from build123d import *

# Parameters (mm, degrees)
SKETCH2_W           = 29.3
SKETCH2_H           = 18.3
BOSS_EXTRUDE1_DEPTH = 1.6
SKETCH3_R           = 4
BOSS_EXTRUDE2_DEPTH = 1
SKETCH4_R           = 3.125
BOSS_EXTRUDE3_DEPTH = 1.6
SKETCH5_R           = 3.9
BOSS_EXTRUDE4_DEPTH = 8.5


with BuildPart() as part:
    # Sketch2 → Boss-Extrude1 (new body)
    with BuildSketch(Plane(origin=(0, 0, 0), x_dir=(1, 0, 0), z_dir=(0, 1, 0))):
        with Locations((14.65, 9.15)):
            Rectangle(SKETCH2_W, SKETCH2_H)
    extrude(amount=BOSS_EXTRUDE1_DEPTH)

    # Sketch3 → Boss-Extrude2 (add)
    with BuildSketch(Plane(origin=(29.3, 0, 0), x_dir=(0, 0, -1), z_dir=(1, 0, 0))):
        with Locations((12.6, 2.1)):
            Circle(SKETCH3_R)
    extrude(amount=BOSS_EXTRUDE2_DEPTH)

    # Sketch4 → Boss-Extrude3 (add)
    with BuildSketch(Plane(origin=(30.3, 0, 0), x_dir=(0, 0, -1), z_dir=(1, 0, 0))):
        with Locations((12.6, 2.1)):
            Circle(SKETCH4_R)
    extrude(amount=BOSS_EXTRUDE3_DEPTH)

    # Sketch5 → Boss-Extrude4 (add)
    with BuildSketch(Plane(origin=(31.9, 0, 0), x_dir=(0, 0, -1), z_dir=(1, 0, 0))):
        with Locations((12.6, 2.1)):
            Circle(SKETCH5_R)
    extrude(amount=BOSS_EXTRUDE4_DEPTH)


solid = part.part
Design review of the part built by this model. Coordinates are the model's own, in mm. A direction names the side the tool comes from. Round coordinates to 2 decimals unless told otherwise and drop trailing zeros. Write each loop counter-clockwise with the first axis right and the second up, starting at its lowest first coordinate (ties: lowest second). Pieces come first, ordered by that corner, then holes. Notation, with made-up numbers: M 59,81 L 74,81 A24 ccw 74,91 Z; hole C 14,15 d3. An arc over 180 degrees is marked long. One line per item, written item: value. Start each with the question number.
1. Take a section at B-B on y = 2.1. State the section outline as (x, z) points (3 decimals), then the cut area to 3 significant figures.
2. Take a section at C-C on x = 26. State the section outline as (y, z) points.
3. Take a section at D-D on x = 33. State the section outline as (y, z) points, then the cut area to 3 significant figures.
4. To check wall thickness, follow probe 1 along X at (y, z) = (3.5, -15.5); probe 2 along Y at (x, z) = (7.5, -8.5); probe 3 along X at (y, z) = (4.5, -12). State the ranges of each line that lie inside material, in increasing order. Write a range as from..to.
5. For faces 4 (the face through (36.09, 2.271, -8.704)), 5 (the face through (14, 1.6, -9)), 6 (the face through (31.9, 0, -10)), 7 (the face through (29.3, -1, -13)), list the 3-axis set-ups (+Z, -Z, +X, -X, +Y, -Y) from which the entire face can be reached by the end or side of a thin tool; tool diameter is ignored.
6. Draft analysis for pull direction X (two halves, no side actions). For faces 1 (the face through (30.3, 0, -10)), 2 (the face through (14, 0, -9)), 3 (the face through (29.3, 3, -13)), state which applies: pulls with the +X half, pulls with the -X half, needs draft (parallel to the pull), parting line crosses it, or undercut.
7. Clearance check with flat-ended pins moving along their axes: P1, Ø1.5, axis at y = -1, z = -14.5, coming from the -X side; P2, Ø2, axis at x = 6.5, z = -5, coming from the -Y side; P3, Ø0.5, axis at y = 0.5, z = -3.5, coming from the +X side. State where each tip first meets the part, or that it passes through.
8. Take a section at A-A on z = -12.6. State the section outline as (x, y) points (3 decimals).
Computed:
1. outline: M 29.3,-16.6 L 30.3,-16.6 L 30.3,-15.725 L 31.9,-15.725 L 31.9,-16.5 L 40.4,-16.5 L 40.4,-8.7 L 31.9,-8.7 L 31.9,-9.475 L 30.3,-9.475 L 30.3,-8.6 L 29.3,-8.6 Z
1. area: 84.3 mm²
2. outline: M 0,-18.3 L 1.6,-18.3 L 1.6,0 L 0,0 Z
3. outline: C 2.1,-12.6 d7.8
3. area: 47.8 mm²
4. probe 1: x = 29.3..30.3, 31.9..40.4
4. probe 2: y = 0..1.6
4. probe 3: x = 29.3..40.4
5. face 4: +X
5. face 5: +Z, -Z, -X, +Y
5. face 6: none
5. face 7: +Z, -Z, -X, -Y
6. face 1: undercut
6. face 2: needs draft
6. face 3: pulls with the -X half
7. P1: stops at x = 29.3
7. P2: stops at y = 0
7. P3: stops at x = 29.3
8. outline: M 0,0 L 29.3,0 L 29.3,-1.9 L 30.3,-1.9 L 30.3,-1.025 L 31.9,-1.025 L 31.9,-1.8 L 40.4,-1.8 L 40.4,6 L 31.9,6 L 31.9,5.225 L 30.3,5.225 L 30.3,6.1 L 29.3,6.1 L 29.3,1.6 L 0,1.6 Z
